```python
from build123d import *
from build123d.topology import SkipClean

# Parameters (mm, degrees)
SKETCH_1_R               = 25
SKETCH_1_R_2             = 12.75
EXTRUDE_1_DEPTH          = 25
CUT_EXTRUDE_1_DEPTH      = 30
CUT_EXTRUDE_1_DEPTH_BACK = 30
SKETCH_2_R               = 2.5
SKETCH_3_W               = 50
SKETCH_3_H               = 90
EXTRUDE_2_DEPTH          = 25
CHAMFER_1_SIZE           = 1
SKETCH_4_R               = 2.9
CUT_EXTRUDE_2_DEPTH      = 20
CHAMFER_2_SIZE           = 1
SKETCH_5_R               = 2.9
CUT_EXTRUDE_3_DEPTH      = 20
CHAMFER_3_SIZE           = 0.5


with BuildPart() as part:
    # 草图1 → 凸台-拉伸1 (new body)
    with BuildSketch(Plane.XY):
        Circle(SKETCH_1_R)
        Circle(SKETCH_1_R_2, mode=Mode.SUBTRACT)
    extrude(amount=EXTRUDE_1_DEPTH)

    # 草图2 → 切除-拉伸1 (cut, two sides: drawn at the far end of the back side and taken through both)
    with BuildSketch(Plane(origin=(0, 0, 0), x_dir=(1, 0, 0), z_dir=(0, 1, 0)).offset(-CUT_EXTRUDE_1_DEPTH_BACK)):
        with Locations(Location((0, -11, 0), (0, 0, 90))):
            Circle(SKETCH_2_R)
    extrude(amount=CUT_EXTRUDE_1_DEPTH + CUT_EXTRUDE_1_DEPTH_BACK, mode=Mode.SUBTRACT)

    # 草图3 → 凸台-拉伸2 (add)
    with BuildSketch(Plane(origin=(0, 0, 0), x_dir=(-1, 0, 0), z_dir=(0, 0, -1))):
        Rectangle(SKETCH_3_W, SKETCH_3_H)
    extrude(amount=EXTRUDE_2_DEPTH)

    # 倒角1
    chamfer_1_edges = [part.edges().sort_by_distance(p)[0] for p in [
        (-25, 0, 25),
        (-12.75, 0, 25),
    ]]
    chamfer(chamfer_1_edges, length=CHAMFER_1_SIZE)

    # 草图4 → 切除-拉伸2 (cut)
    with BuildSketch(Plane(origin=(0, 0, -25), x_dir=(-1, 0, 0), z_dir=(0, 0, -1))):
        with Locations((2, 0)):
            Circle(SKETCH_4_R)
    extrude(amount=-CUT_EXTRUDE_2_DEPTH, mode=Mode.SUBTRACT)

    # 倒角2
    # the kernel refuses this chamfer: 1 mm, written as the material it takes off along each edge
    with BuildSketch(Plane(origin=(25, 0, 0), x_dir=(-0.9996219169112968, 0, 0.02749587661058639), z_dir=(0, 1, 0))) as chamfer_2_piece_1_section:
        Polygon((CHAMFER_2_SIZE * 0.999621916911, -CHAMFER_2_SIZE * 0.0274958766106), (-CHAMFER_2_SIZE * 0.0274958766106, -CHAMFER_2_SIZE * 0.999621916911), (0, 0), align=None)
    chamfer_2_piece_1 = extrude(amount=47.571682988, mode=Mode.PRIVATE)
    chamfer_2_piece_1 = chamfer_2_piece_1 - Plane(origin=(0, 0, -0.337643677), x_dir=(1, 0, 0), z_dir=(0, 0, -1)) * Cylinder(25, 100, mode=Mode.PRIVATE)
    add(chamfer_2_piece_1, mode=Mode.SUBTRACT)
    with BuildSketch(Plane(origin=(25, -47.571682988, 0), x_dir=(-0.9996219169112968, 0, 0.02749587661058639), z_dir=(0, 1, 0))) as chamfer_2_piece_2_section:
        Polygon((CHAMFER_2_SIZE * 0.999621916911, -CHAMFER_2_SIZE * 0.0274958766106), (-CHAMFER_2_SIZE * 0.0274958766106, -CHAMFER_2_SIZE * 0.999621916911), (0, 0), align=None)
    chamfer_2_piece_2 = extrude(amount=47.571682988, mode=Mode.PRIVATE)
    chamfer_2_piece_2 = chamfer_2_piece_2 - Plane(origin=(0, 0, -0.337643676), x_dir=(1, 0, 0), z_dir=(0, 0, -1)) * Cylinder(25, 100, mode=Mode.PRIVATE)
    add(chamfer_2_piece_2, mode=Mode.SUBTRACT)
    with BuildSketch(Plane(origin=(-27.571682988, -45, 0), x_dir=(0, 0.9996219169112968, 0.027495876610586292), z_dir=(1, 0, 0)), Plane(origin=(27.571682988, 45, 0), x_dir=(0, -0.9996219169112968, 0.027495876610586292), z_dir=(-1, 0, 0)), Plane(origin=(-27.571682988, -45, -25), x_dir=(0, -0.0274958766105891, 0.9996219169112968), z_dir=(1, 0, 0)), Plane(origin=(27.571682988, 45, -25), x_dir=(0, 0.0274958766105891, 0.9996219169112968), z_dir=(-1, 0, 0))) as chamfer_2_piece_3:
        Polygon((CHAMFER_2_SIZE * 0.999621916911, -CHAMFER_2_SIZE * 0.0274958766106), (-CHAMFER_2_SIZE * 0.0274958766106, -CHAMFER_2_SIZE * 0.999621916911), (0, 0), align=None)
    extrude(amount=55.143365976, mode=Mode.SUBTRACT)
    with BuildSketch(Plane(origin=(-25, -1.3e-08, 0), x_dir=(0.9996219169112968, 0, 0.02749587661058639), z_dir=(0, -1, 0))) as chamfer_2_piece_4_section:
        Polygon((CHAMFER_2_SIZE * 0.999621916911, -CHAMFER_2_SIZE * 0.0274958766106), (-CHAMFER_2_SIZE * 0.0274958766106, -CHAMFER_2_SIZE * 0.999621916911), (0, 0), align=None)
    chamfer_2_piece_4 = extrude(amount=47.571682975, mode=Mode.PRIVATE)
    chamfer_2_piece_4 = chamfer_2_piece_4 - Plane(origin=(0, 0, -0.337643677), x_dir=(1, 0, 0), z_dir=(0, 0, -1)) * Cylinder(25, 100, mode=Mode.PRIVATE)
    add(chamfer_2_piece_4, mode=Mode.SUBTRACT)
    with BuildSketch(Plane(origin=(-25, 47.571682988, 0), x_dir=(0.9996219169112968, 0, 0.02749587661058639), z_dir=(0, -1, 0))) as chamfer_2_piece_5_section:
        Polygon((CHAMFER_2_SIZE * 0.999621916911, -CHAMFER_2_SIZE * 0.0274958766106), (-CHAMFER_2_SIZE * 0.0274958766106, -CHAMFER_2_SIZE * 0.999621916911), (0, 0), align=None)
    chamfer_2_piece_5 = extrude(amount=47.571683001, mode=Mode.PRIVATE)
    chamfer_2_piece_5 = chamfer_2_piece_5 - Plane(origin=(0, 0, -0.337643677), x_dir=(1, 0, 0), z_dir=(0, 0, -1)) * Cylinder(25, 100, mode=Mode.PRIVATE)
    add(chamfer_2_piece_5, mode=Mode.SUBTRACT)
    with BuildSketch(Plane(origin=(25, -47.571682988, -25), x_dir=(0.027495876610585647, 0, 0.9996219169112968), z_dir=(0, 1, 0)), Plane(origin=(-25, 47.571682988, -25), x_dir=(-0.027495876610585647, 0, 0.9996219169112968), z_dir=(0, -1, 0))) as chamfer_2_piece_6:
        Polygon((CHAMFER_2_SIZE * 0.999621916911, -CHAMFER_2_SIZE * 0.0274958766106), (-CHAMFER_2_SIZE * 0.0274958766106, -CHAMFER_2_SIZE * 0.999621916911), (0, 0), align=None)
    extrude(amount=95.143365976, mode=Mode.SUBTRACT)
    with BuildSketch(Plane(origin=(-2, 0, -25), x_dir=(-1, 0, 0), z_dir=(0, -1, 0))) as chamfer_2_piece_7:
        Polygon((2.9 + CHAMFER_2_SIZE, 0), (2.9, -CHAMFER_2_SIZE), (2.9, 0), align=None)
    revolve(axis=Axis((-2, 0, -25), (0, 0, -1)), mode=Mode.SUBTRACT)

    # 草图5 → 切除-拉伸3 (cut)
    with SkipClean():  # the faces are left unmerged after this step: merging them gives an invalid solid
        with BuildSketch(Plane(origin=(0, 0, -25), x_dir=(-1, 0, 0), z_dir=(0, 0, -1))):
            with Locations((2, 34)):
                Circle(SKETCH_5_R)
            with Locations((2, -34)):
                Circle(SKETCH_5_R)
        extrude(amount=-CUT_EXTRUDE_3_DEPTH, mode=Mode.SUBTRACT)

    # 倒角3
    chamfer_3_edges = [part.edges().sort_by_distance(p)[0] for p in [
        (0.9, 34, -25),
        (0.9, -34, -25),
    ]]
    chamfer(chamfer_3_edges, length=CHAMFER_3_SIZE)


solid = part.part
```
CAD build for the part. Positions are in the model's coordinates, mm. A direction names the side the tool comes from. Coordinates: 2 decimals unless noted, no trailing zeros. Order: outer loops, then holes, each group sorted by start corner. A loop starts at its lowest first (then second) coordinate and runs counter-clockwise, first axis right, second up. Notation, with made-up numbers: M 23,89.5 L 59,89.5 A11 cw 59,105.5 Z; hole C 61.5,-19 d11. An arc over 180 degrees is marked long. Write each question's results on one line, items separated by ' | '. Start each with the question number.
Q1. Flat gauge pins, fed straight in: P1, Ø4.5, axis at x = -3, y = 1, coming from the -Z side; P2, Ø3, axis at x = -5.5, z = 10.5, coming from the +Y side; P3, Ø5, axis at x = -7.5, y = -24, coming from the +Z side; P4, Ø4.5, axis at x = -1.5, y = -33.5, coming from the -Z side. Where does each tip first touch, or does it go through?
Q2. Cut at A-A (y = -34). List the corners of the cut face in (x, z), then the cut area to 3 significant figures.
Q3. Which spindle directions (+Z, -Z, +X, -X, +Y, -Y) get a long thin tool onto all of the face, cutting with end or side? Do faces 1 (the cylindrical face through (-0.1, -18.8, 13.5)), 2 (the flat face through (-2, -34, -5)), 3 (the flat face through (0, 0, 0)). Say none if no direction does.
Q4. Drill centre lines: probe 1 along Y at (x, z) = (-2, -12.75); probe 2 along Z at (x, y) = (1, 11); probe 3 along Y at (x, z) = (-1, 17). Where is each one in solid material? Low to high. Write a range as from..to.
Q5. Pull direction Y, two halves, no side cores. Call faces 4 (the flat face through (-2, 34, -5)), 5 (the flat face through (0, 45, -12)), 6 (the flat face through (0, 34, 0)), 7 (the flat face through (0, -45, -12)): +Y half, -Y half, draft (parallel to the pull), parting line (faces both ways), or undercut.
Q6. Cut at C-C (y = 39.5). List the corners of the cut face in (x, z), then the cut area to 3 significant figures.
Q7. Cut at B-B (z = 6.5). List the corners of the cut face in (x, y).
Found:
1) P1: z = -24.76 | P2: y = 24.68 | P3: z = 25 | P4: z = -24.56
2) outline: M -25,-24 L -24,-25 L -5.4,-25 L -4.9,-24.5 L -4.9,-5 L 0.9,-5 L 0.9,-24.5 L 1.4,-25 L 24,-25 L 25,-24 L 25,-1 L 24,0 L -24,0 L -25,-1 Z | area: 1,130 mm²
3) face 1: +Y, -Y | face 2: -Z | face 3: +Z
4) probe 1: -45..-36.9, -31.1..-2.9, 2.9..31.1, 36.9..45 | probe 2: -25..0 | probe 3: -24.98..-12.71, 12.71..24.98
5) face 4: undercut | face 5: +Y half | face 6: draft | face 7: -Y half
6) outline: M -25,-24 L -24,-25 L 24,-25 L 25,-24 L 25,-1 L 24,0 L -24,0 L -25,-1 Z | area: 1,250 mm²
7) outline: C 0,0 d50; hole C 0,0 d25.5
